from build123d import *

# Parameters (mm, degrees)
F0_R         = 10
F1_DEPTH     = 1.4
F2_R         = 5.5
F3_DEPTH     = 1.4
F4_R         = 4.1
F4_R_2       = 2.5
F5_DEPTH     = 4.2
F7_DEPTH     = 1.4
F8_T4_DEPTH  = 2.85
F8_S5_R      = 4.1
F8_T6_DEPTH  = 3
F8_S7_R      = 2.5
F8_T8_DEPTH  = 3
F8_T12_DEPTH = 2.85
F8_S13_R     = 4.1
F8_T14_DEPTH = 3
F8_S15_R     = 2.5
F8_T16_DEPTH = 3
F8_T20_DEPTH = 2.85
F8_S21_R     = 4.1
F8_T22_DEPTH = 3
F8_S23_R     = 2.5
F8_T24_DEPTH = 3
F8_T28_DEPTH = 2.85
F8_S29_R     = 4.1
F8_T30_DEPTH = 3
F8_S31_R     = 2.5
F8_T32_DEPTH = 3
F8_T36_DEPTH = 2.85
F8_S37_R     = 4.1
F8_T38_DEPTH = 3
F8_S39_R     = 2.5
F8_T40_DEPTH = 3
F8_T44_DEPTH = 2.85
F8_S45_R     = 4.1
F8_T46_DEPTH = 3
F8_S47_R     = 2.5
F8_T48_DEPTH = 3
F8_T52_DEPTH = 2.85
F8_S53_R     = 4.1
F8_T54_DEPTH = 3
F8_S55_R     = 2.5
F8_T56_DEPTH = 3
F8_T60_DEPTH = 2.85
F8_S61_R     = 4.1
F8_T62_DEPTH = 3
F8_S63_R     = 2.5
F8_T64_DEPTH = 3
F8_T65_DEPTH = 2.85
F8_T67_DEPTH = 2.85
F8_T69_DEPTH = 2.85
F8_T71_DEPTH = 2.85
F8_T73_DEPTH = 2.85
F8_T75_DEPTH = 2.85
F8_T77_DEPTH = 2.85
F8_T79_DEPTH = 2.85


# Not quite as in the source:
# - a fillet or chamfer that OpenCascade refuses, or shapes differently, is made with other operations: its cross-section is extruded or revolved along the edge and cut away or added


with BuildPart() as f1:
    # F0 (on Top) → F1 (new body)
    with BuildSketch(Plane.XY):
        Circle(F0_R)
    extrude(amount=F1_DEPTH)

    # F2 (on face) → F3 (join)
    with BuildSketch(Plane.XY.offset(1.4)):
        Circle(F2_R)
    extrude(amount=F3_DEPTH)

    # F4 (on face) → F5 (join)
    with BuildSketch(Plane.XY.offset(2.8)):
        Circle(F4_R)
        Circle(F4_R_2, mode=Mode.SUBTRACT)
    extrude(amount=F5_DEPTH)

    # F6 (on face) → F7 (cut)
    with BuildSketch(Plane.XY.offset(7)):
        with BuildLine():
            Line((0, -2.5), (0, -4.1))
            ThreePointArc((0, -4.1), (1.5690020727, -3.7879060833), (2.8991378029, -2.8991378029))
            Line((2.8991378029, -2.8991378029), (1.767766953, -1.767766953))
            ThreePointArc((1.767766953, -1.767766953), (0.9567085809, -2.3096988313), (0, -2.5))
        make_face()
        with BuildLine():
            ThreePointArc((-4.1, 0), (-3.7879060833, -1.5690020727), (-2.8991378029, -2.8991378029))
            Line((-2.8991378029, -2.8991378029), (-1.767766953, -1.767766953))
            ThreePointArc((-1.767766953, -1.767766953), (-2.3096988313, -0.9567085809), (-2.5, 0))
            Line((-2.5, 0), (-4.1, 0))
        make_face()
        with BuildLine():
            Line((2.5, 0), (4.1, 0))
            ThreePointArc((4.1, 0), (3.7879060833, 1.5690020727), (2.8991378029, 2.8991378029))
            Line((2.8991378029, 2.8991378029), (1.767766953, 1.767766953))
            ThreePointArc((1.767766953, 1.767766953), (2.3096988313, 0.9567085809), (2.5, 0))
        make_face()
        with BuildLine():
            ThreePointArc((-1.767766953, 1.767766953), (-0.9567085809, 2.3096988313), (0, 2.5))
            Line((0, 2.5), (0, 4.1))
            ThreePointArc((0, 4.1), (-1.5690020727, 3.7879060833), (-2.8991378029, 2.8991378029))
            Line((-2.8991378029, 2.8991378029), (-1.767766953, 1.767766953))
        make_face()
    extrude(amount=-F7_DEPTH, mode=Mode.SUBTRACT)

    # F8: fillet of radius 0.25 on 16 edges, made by hand


with BuildPart() as f8_tool2:
    # F8_s3 → F8_t4 (new body)
    with BuildSketch(Plane.YZ.offset(-1.875)):
        with BuildLine():
            ThreePointArc((-0.25, 5.6), (-0.0732233047, 5.6732233047), (0, 5.85))
            Line((0, 5.85), (0, 5.6))
            Line((0, 5.6), (-0.25, 5.6))
        make_face()
    extrude(amount=-F8_T4_DEPTH)

    # F8_s5 → F8_t6 (intersect, symmetric)
    with BuildSketch(Plane.XY.offset(5.7)):
        Circle(F8_S5_R)
    extrude(amount=F8_T6_DEPTH, both=True, mode=Mode.INTERSECT)

    # F8_s7 → F8_t8 (cut, symmetric)
    with BuildSketch(Plane.XY.offset(5.7)):
        Circle(F8_S7_R)
    extrude(amount=F8_T8_DEPTH, both=True, mode=Mode.SUBTRACT)


with BuildPart() as f1_1:
    add(f1.part)

    # F8_t1: union F8_tool2
    add(f8_tool2.part)


with BuildPart() as f8_tool10:
    # F8_s11 → F8_t12 (new body)
    with BuildSketch(Plane.XZ.offset(-1.875)):
        with BuildLine():
            ThreePointArc((-0.25, 5.6), (-0.0732233047, 5.6732233047), (0, 5.85))
            Line((0, 5.85), (0, 5.6))
            Line((0, 5.6), (-0.25, 5.6))
        make_face()
    extrude(amount=-F8_T12_DEPTH)

    # F8_s13 → F8_t14 (intersect, symmetric)
    with BuildSketch(Plane.XY.offset(5.7)):
        Circle(F8_S13_R)
    extrude(amount=F8_T14_DEPTH, both=True, mode=Mode.INTERSECT)

    # F8_s15 → F8_t16 (cut, symmetric)
    with BuildSketch(Plane.XY.offset(5.7)):
        Circle(F8_S15_R)
    extrude(amount=F8_T16_DEPTH, both=True, mode=Mode.SUBTRACT)


with BuildPart() as f1_2:
    add(f1_1.part)

    # F8_t9: union F8_tool10
    add(f8_tool10.part)


with BuildPart() as f8_tool18:
    # F8_s19 → F8_t20 (new body)
    with BuildSketch(Plane(origin=(3.3410795411, -3.3410795411, 0), x_dir=(0, 0, 1), z_dir=(-0.7071067812, 0.7071067812, 0))):
        with BuildLine():
            ThreePointArc((5.85, 0), (5.6732233047, -0.0732233047), (5.6, -0.25))
            Line((5.6, -0.25), (5.6, 0))
            Line((5.6, 0), (5.85, 0))
        make_face()
    extrude(amount=F8_T20_DEPTH)

    # F8_s21 → F8_t22 (intersect, symmetric)
    with BuildSketch(Plane.XY.offset(5.7)):
        Circle(F8_S21_R)
    extrude(amount=F8_T22_DEPTH, both=True, mode=Mode.INTERSECT)

    # F8_s23 → F8_t24 (cut, symmetric)
    with BuildSketch(Plane.XY.offset(5.7)):
        Circle(F8_S23_R)
    extrude(amount=F8_T24_DEPTH, both=True, mode=Mode.SUBTRACT)


with BuildPart() as f1_3:
    add(f1_2.part)

    # F8_t17: union F8_tool18
    add(f8_tool18.part)


with BuildPart() as f8_tool26:
    # F8_s27 → F8_t28 (new body)
    with BuildSketch(Plane.YZ.offset(1.875)):
        with BuildLine():
            ThreePointArc((0, 5.85), (0.0732233047, 5.6732233047), (0.25, 5.6))
            Line((0.25, 5.6), (0, 5.6))
            Line((0, 5.6), (0, 5.85))
        make_face()
    extrude(amount=F8_T28_DEPTH)

    # F8_s29 → F8_t30 (intersect, symmetric)
    with BuildSketch(Plane.XY.offset(5.7)):
        Circle(F8_S29_R)
    extrude(amount=F8_T30_DEPTH, both=True, mode=Mode.INTERSECT)

    # F8_s31 → F8_t32 (cut, symmetric)
    with BuildSketch(Plane.XY.offset(5.7)):
        Circle(F8_S31_R)
    extrude(amount=F8_T32_DEPTH, both=True, mode=Mode.SUBTRACT)


with BuildPart() as f1_4:
    add(f1_3.part)

    # F8_t25: union F8_tool26
    add(f8_tool26.part)


with BuildPart() as f8_tool34:
    # F8_s35 → F8_t36 (new body)
    with BuildSketch(Plane(origin=(-3.3410795411, -3.3410795411, 0), x_dir=(0, 0, 1), z_dir=(0.7071067812, 0.7071067812, 0))):
        with BuildLine():
            ThreePointArc((5.85, 0), (5.6732233047, -0.0732233047), (5.6, -0.25))
            Line((5.6, -0.25), (5.6, 0))
            Line((5.6, 0), (5.85, 0))
        make_face()
    extrude(amount=F8_T36_DEPTH)

    # F8_s37 → F8_t38 (intersect, symmetric)
    with BuildSketch(Plane.XY.offset(5.7)):
        Circle(F8_S37_R)
    extrude(amount=F8_T38_DEPTH, both=True, mode=Mode.INTERSECT)

    # F8_s39 → F8_t40 (cut, symmetric)
    with BuildSketch(Plane.XY.offset(5.7)):
        Circle(F8_S39_R)
    extrude(amount=F8_T40_DEPTH, both=True, mode=Mode.SUBTRACT)


with BuildPart() as f1_5:
    add(f1_4.part)

    # F8_t33: union F8_tool34
    add(f8_tool34.part)


with BuildPart() as f8_tool42:
    # F8_s43 → F8_t44 (new body)
    with BuildSketch(Plane(origin=(-3.3410795411, 3.3410795411, 0), x_dir=(0, 0, 1), z_dir=(0.7071067812, -0.7071067812, 0))):
        with BuildLine():
            ThreePointArc((5.85, 0), (5.6732233047, -0.0732233047), (5.6, -0.25))
            Line((5.6, -0.25), (5.6, 0))
            Line((5.6, 0), (5.85, 0))
        make_face()
    extrude(amount=F8_T44_DEPTH)

    # F8_s45 → F8_t46 (intersect, symmetric)
    with BuildSketch(Plane.XY.offset(5.7)):
        Circle(F8_S45_R)
    extrude(amount=F8_T46_DEPTH, both=True, mode=Mode.INTERSECT)

    # F8_s47 → F8_t48 (cut, symmetric)
    with BuildSketch(Plane.XY.offset(5.7)):
        Circle(F8_S47_R)
    extrude(amount=F8_T48_DEPTH, both=True, mode=Mode.SUBTRACT)


with BuildPart() as f1_6:
    add(f1_5.part)

    # F8_t41: union F8_tool42
    add(f8_tool42.part)


with BuildPart() as f8_tool50:
    # F8_s51 → F8_t52 (new body)
    with BuildSketch(Plane.XZ.offset(1.875)):
        with BuildLine():
            ThreePointArc((0.25, 5.6), (0.0732233047, 5.6732233047), (0, 5.85))
            Line((0, 5.85), (0, 5.6))
            Line((0, 5.6), (0.25, 5.6))
        make_face()
    extrude(amount=F8_T52_DEPTH)

    # F8_s53 → F8_t54 (intersect, symmetric)
    with BuildSketch(Plane.XY.offset(5.7)):
        Circle(F8_S53_R)
    extrude(amount=F8_T54_DEPTH, both=True, mode=Mode.INTERSECT)

    # F8_s55 → F8_t56 (cut, symmetric)
    with BuildSketch(Plane.XY.offset(5.7)):
        Circle(F8_S55_R)
    extrude(amount=F8_T56_DEPTH, both=True, mode=Mode.SUBTRACT)


with BuildPart() as f1_7:
    add(f1_6.part)

    # F8_t49: union F8_tool50
    add(f8_tool50.part)


with BuildPart() as f8_tool58:
    # F8_s59 → F8_t60 (new body)
    with BuildSketch(Plane(origin=(3.3410795411, 3.3410795411, 0), x_dir=(0, 0, 1), z_dir=(-0.7071067812, -0.7071067812, 0))):
        with BuildLine():
            ThreePointArc((5.85, 0), (5.6732233047, -0.0732233047), (5.6, -0.25))
            Line((5.6, -0.25), (5.6, 0))
            Line((5.6, 0), (5.85, 0))
        make_face()
    extrude(amount=F8_T60_DEPTH)

    # F8_s61 → F8_t62 (intersect, symmetric)
    with BuildSketch(Plane.XY.offset(5.7)):
        Circle(F8_S61_R)
    extrude(amount=F8_T62_DEPTH, both=True, mode=Mode.INTERSECT)

    # F8_s63 → F8_t64 (cut, symmetric)
    with BuildSketch(Plane.XY.offset(5.7)):
        Circle(F8_S63_R)
    extrude(amount=F8_T64_DEPTH, both=True, mode=Mode.SUBTRACT)


with BuildPart() as f1_8:
    add(f1_7.part)

    # F8_t57: union F8_tool58
    add(f8_tool58.part)

    # F8_s66 → F8_t65 (cut)
    with BuildSketch(Plane.YZ.offset(-4.725)):
        with BuildLine():
            ThreePointArc((0, 6.75), (0.0732233047, 6.9267766953), (0.25, 7))
            Line((0.25, 7), (0, 7))
            Line((0, 7), (0, 6.75))
        make_face()
    extrude(amount=F8_T65_DEPTH, mode=Mode.SUBTRACT)

    # F8_s68 → F8_t67 (cut)
    with BuildSketch(Plane(origin=(-3.3410795411, 3.3410795411, 0), x_dir=(0, 0, 1), z_dir=(0.7071067812, -0.7071067812, 0))):
        with BuildLine():
            ThreePointArc((7, 0.25), (6.9267766953, 0.0732233047), (6.75, 0))
            Line((6.75, 0), (7, 0))
            Line((7, 0), (7, 0.25))
        make_face()
    extrude(amount=F8_T67_DEPTH, mode=Mode.SUBTRACT)

    # F8_s70 → F8_t69 (cut)
    with BuildSketch(Plane.XZ.offset(1.875)):
        with BuildLine():
            ThreePointArc((0, 6.75), (-0.0732233047, 6.9267766953), (-0.25, 7))
            Line((-0.25, 7), (0, 7))
            Line((0, 7), (0, 6.75))
        make_face()
    extrude(amount=F8_T69_DEPTH, mode=Mode.SUBTRACT)

    # F8_s72 → F8_t71 (cut)
    with BuildSketch(Plane(origin=(-3.3410795411, -3.3410795411, 0), x_dir=(0, 0, 1), z_dir=(0.7071067812, 0.7071067812, 0))):
        with BuildLine():
            ThreePointArc((7, 0.25), (6.9267766953, 0.0732233047), (6.75, 0))
            Line((6.75, 0), (7, 0))
            Line((7, 0), (7, 0.25))
        make_face()
    extrude(amount=F8_T71_DEPTH, mode=Mode.SUBTRACT)

    # F8_s74 → F8_t73 (cut)
    with BuildSketch(Plane.YZ.offset(1.875)):
        with BuildLine():
            ThreePointArc((0, 6.75), (-0.0732233047, 6.9267766953), (-0.25, 7))
            Line((-0.25, 7), (0, 7))
            Line((0, 7), (0, 6.75))
        make_face()
    extrude(amount=F8_T73_DEPTH, mode=Mode.SUBTRACT)

    # F8_s76 → F8_t75 (cut)
    with BuildSketch(Plane(origin=(3.3410795411, -3.3410795411, 0), x_dir=(0, 0, 1), z_dir=(-0.7071067812, 0.7071067812, 0))):
        with BuildLine():
            ThreePointArc((7, 0.25), (6.9267766953, 0.0732233047), (6.75, 0))
            Line((6.75, 0), (7, 0))
            Line((7, 0), (7, 0.25))
        make_face()
    extrude(amount=F8_T75_DEPTH, mode=Mode.SUBTRACT)

    # F8_s78 → F8_t77 (cut)
    with BuildSketch(Plane.XZ.offset(-4.725)):
        with BuildLine():
            ThreePointArc((0, 6.75), (0.0732233047, 6.9267766953), (0.25, 7))
            Line((0.25, 7), (0, 7))
            Line((0, 7), (0, 6.75))
        make_face()
    extrude(amount=F8_T77_DEPTH, mode=Mode.SUBTRACT)

    # F8_s80 → F8_t79 (cut)
    with BuildSketch(Plane(origin=(3.3410795411, 3.3410795411, 0), x_dir=(0, 0, 1), z_dir=(-0.7071067812, -0.7071067812, 0))):
        with BuildLine():
            ThreePointArc((7, 0.25), (6.9267766953, 0.0732233047), (6.75, 0))
            Line((6.75, 0), (7, 0))
            Line((7, 0), (7, 0.25))
        make_face()
    extrude(amount=F8_T79_DEPTH, mode=Mode.SUBTRACT)


solid = f1_8.part
The listing builds one solid part. Answer for the finished solid, in the listing's coordinates (mm). A direction names the side the tool comes from. Coordinates: 2 decimals unless noted, no trailing zeros. Write each loop counter-clockwise with the first axis right and the second up, starting at its lowest first coordinate (ties: lowest second). Pieces come first, ordered by that corner, then holes. Notation, with made-up numbers: (40, -17.5) -> (48, -17.5) arc R29 ccw to (48, 16.5) -> close; hole circle Ø8 at (-1.5, 49.25). An arc over 180 degrees is marked (long way). One line per question, with ' | ' between items.
1. For a pull along Y with two mould halves and no side action, classify faces 4 (the flat face through (-2, -2, 6)), 5 (the flat face through (0, 3, 6)), 6 (the flat face through (-2, 2, 6)) as released by +Y, released by -Y, zero draft, split by the parting line, or undercut.
Verdict:
face 4: undercut | face 5: zero draft | face 6: released by +Y
2. Section A-A (z = 4.5) is taken. Determine the outline of the cut face in (x, y), and give its area (3 significant figures).
Verdict:
outline: circle Ø8.2 at (0, 0); hole circle Ø5 at (0, 0) | area: 33.2 mm^2
3. Section C-C (x = -0.5) is taken. Determine the outline of the cut face in (y, z), and give its area (3 significant figures).
Verdict:
outline: (-9.99, 0) -> (9.99, 0) -> (9.99, 1.4) -> (5.48, 1.4) -> (5.48, 2.8) -> (4.07, 2.8) -> (4.07, 5.6) -> (2.45, 5.6) -> (2.45, 2.8) -> (-2.45, 2.8) -> (-2.45, 7) -> (-4.07, 7) -> (-4.07, 2.8) -> (-5.48, 2.8) -> (-5.48, 1.4) -> (-9.99, 1.4) -> close | area: 54.6 mm^2
4. Which of the six approach directions +Z, -Z, +X, -X, +Y, -Y give full straight-line access (tool end or side, diameter ignored) to faces 1 (the flat face through (2, -2, 6)), 2 (the flat face through (-3, -1, 5.6)), 3 (the cylindrical face through (-1.19, -5.37, 2.09))?
Verdict:
face 1: +Z, -Y | face 2: +Z, -X | face 3: +Z
5. Given pin 1 Ø1.1 at (x, y) = (1, -3.5) entering from +Z; pin 2 Ø1.5 at (x, z) = (-0.5, 5.5) entering from +Y; pin 3 Ø4 at (y, z) = (2.5, 5) entering from -X; pin 4 Ø3 at (y, z) = (-6.5, 5) entering from +X, each flat-ended and moving along its own axis, determine where each tip first touches the part or whether it passes through.
Verdict:
pin 1: stops at z = 5.6 | pin 2: stops at y = 4.1 | pin 3: stops at x = -4.07 | pin 4: passes through
6. Straight lines are drawn through the part: line 1 (Y direction, x = 0, z = 4.55); line 2 (Z direction, x = 4.5, y = 7.75); line 3 (X direction, y = -3.25, z = 3.75). For each, find the intervals that lie inside material, in ascending order.
Verdict:
line 1: y = -4.1 to -2.5, 2.5 to 4.1 | line 2: z = 0 to 1.4 | line 3: x = -2.5 to 2.5
7. Section D-D (y = 7.5) is taken. Determine the outline of the cut face in (x, z).
Verdict:
outline: (-6.61, 0) -> (6.61, 0) -> (6.61, 1.4) -> (-6.61, 1.4) -> close
8. Section B-B (z = 2.5) is taken. Determine the outline of the cut face in (x, y), and give its area (3 significant figures).
Verdict:
outline: circle Ø11 at (0, 0) | area: 95.0 mm^2
